Design review of the part built by this model. Coordinates are the model's own, in mm. A direction names the side the tool comes from. Coordinates: 2 decimals unless noted, no trailing zeros. Order: outer loops, then holes, each group sorted by start corner. A loop starts at its lowest first (then second) coordinate and runs counter-clockwise, first axis right, second up. Notation, with made-up numbers: M -39,-31 L -9,-31 A20 ccw -9,-11 Z; hole C 17,73.25 d6. An arc over 180 degrees is marked long. Use CSV: the item, a comma, the result in double quotes.
```python
from build123d import *

# Parameters (mm, degrees)
SKETCH_1_W               = 62
SKETCH_1_H               = 24
SKETCH_1_R               = 4.5
EXTRUDE_1_DEPTH          = 8
EXTRUDE_2_DEPTH          = 14
CUT_EXTRUDE_2_DEPTH      = 8
CUT_EXTRUDE_3_DEPTH      = 68.453687816
CUT_EXTRUDE_3_DEPTH_BACK = 68.453687816
SKETCH_6_R               = 4


with BuildPart() as part:
    # 草图1 → 凸台-拉伸1 (new body)
    with BuildSketch(Plane.XY):
        Rectangle(SKETCH_1_W, SKETCH_1_H)
        with Locations((-22.5, 0)):
            Circle(SKETCH_1_R, mode=Mode.SUBTRACT)
        with Locations(Location((22.5, 0, 0), (0, 0, 180))):
            Circle(SKETCH_1_R, mode=Mode.SUBTRACT)
    extrude(amount=EXTRUDE_1_DEPTH)

    # 草图2 → 凸台-拉伸2 (add, symmetric)
    with BuildSketch(Plane(origin=(0, 0, 0), x_dir=(0, 0, -1), z_dir=(1, 0, 0))):
        with BuildLine():
            Line((-8, 12), (-14, 12))
            Line((-14, 12), (-35.191485533, -18.26418578))
            ThreePointArc((-35.191485533, -18.26418578), (-32.73581422, -32.191485533), (-18.808514467, -29.73581422))
            Line((-18.808514467, -29.73581422), (-8, -12))
            Line((-8, -12), (0, -12))
            Line((0, -12), (0, 12))
            Line((0, 12), (-8, 12))
        make_face()
    extrude(amount=EXTRUDE_2_DEPTH, both=True)

    # 草图5 → 切除-拉伸2 (cut, symmetric)
    with BuildSketch(Plane(origin=(0, 0, 0), x_dir=(0, 0, -1), z_dir=(1, 0, 0))):
        with BuildLine():
            Line((-18.808514467, -29.73581422), (-8, -12))
            Line((-8, -12), (-8, 12))
            Line((-8, 12), (-14, 12))
            Line((-14, 12), (-35.191485533, -18.26418578))
            ThreePointArc((-35.191485533, -18.26418578), (-32.73581422, -32.191485533), (-18.808514467, -29.73581422))
        make_face()
    extrude(amount=CUT_EXTRUDE_2_DEPTH, both=True, mode=Mode.SUBTRACT)

    # 草图6 → 切除-拉伸3 (cut, two sides: drawn at the far end of the back side and taken through both)
    with BuildSketch(Plane(origin=(14, 0, 0), x_dir=(0, 0, -1), z_dir=(1, 0, 0)).offset(-CUT_EXTRUDE_3_DEPTH_BACK)):
        with Locations((-27, -24)):
            Circle(SKETCH_6_R)
    extrude(amount=CUT_EXTRUDE_3_DEPTH + CUT_EXTRUDE_3_DEPTH_BACK, mode=Mode.SUBTRACT)


solid = part.part
```
(1) Wall thickness on probe 1 along X at (y, z) = (0.5, 10); probe 2 along X at (y, z) = (4, 7.5); probe 3 along Z at (x, y) = (-23, -10.5): over which ranges is each line inside the solid? List them lowest first.
The answers:
probe 1,"x = -14 to -8, 8 to 14"
probe 2,"x = -31 to -24.56, -20.44 to 20.44, 24.56 to 31"
probe 3,"z = 0 to 8"
(2) The part is to be moulded in two halves that separate along X. For faces 1 (the face through (-14, -11, 19)), 2 (the face through (-11.04, -21.3, 29.95)), 3 (the face through (-8, -11, 19)), 4 (the face through (-27, 0, 4)), say which applies: pulls with the +X half, pulls with the -X half, needs draft (parallel to the pull), parting line crosses it, or undercut.
The answers:
face 1,"pulls with the -X half"
face 2,"needs draft"
face 3,"undercut"
face 4,"undercut"
(3) For faces 5 (the face through (0, 0, 8)), 6 (the face through (27, 0, 4)), 7 (the face through (14, -11, 19)), list the 3-axis set-ups (+Z, -Z, +X, -X, +Y, -Y) from which the entire face can be reached by the end or side of a thin tool; tool diameter is ignored.
The answers:
face 5,"+Z, +Y, -Y"
face 6,"+Z, -Z"
face 7,"+Z, +X, +Y, -Y"
(4) Add section B-B on z = 19.5. State the section outline as (x, y) points.
The answers:
outline,"M -14,-30.61 L -8,-30.61 L -8,4.15 L -14,4.15 Z; M 8,-30.61 L 14,-30.61 L 14,4.15 L 8,4.15 Z"
(5) Add section A-A on x = -22.5. State the section outline as (y, z) points.
The answers:
outline,"M -12,0 L -4.5,0 L -4.5,8 L -12,8 Z; M 4.5,0 L 12,0 L 12,8 L 4.5,8 Z"
(6) Add section D-D on z = 5. State the section outline as (x, y) points, and give its area (3 significant figures).
The answers:
outline,"M -31,-12 L 31,-12 L 31,12 L -31,12 Z; hole C -22.5,0 d9; hole C 22.5,0 d9"
area,"1,360 mm2"
(7) Add section C-C on y = 0. State the section outline as (x, z) points.
The answers:
outline,"M -31,0 L -27,0 L -27,8 L -31,8 Z; M -18,0 L 18,0 L 18,8 L 14,8 L 14,22.4 L 8,22.4 L 8,8 L -8,8 L -8,22.4 L -14,22.4 L -14,8 L -18,8 Z; M 27,0 L 31,0 L 31,8 L 27,8 Z"
(8) Clearance check with flat-ended pins moving along their axes: P1, Ø5, axis at x = 6, y = -26.5, coming from the -Z side; P2, Ø8.5, axis at y = -14, z = 23, coming from the -X side; P3, Ø8, axis at x = -9.5, y = -2.5, coming from the +Z side. State where each tip first meets the part, or that it passes through.
The answers:
P1,"stops at z = 15.92"
P2,"stops at x = -14"
P3,"stops at z = 26.95"
